```python
from build123d import *

# Parameters (mm, degrees)
F0_W     = 16
F0_H     = 46
F0_R     = 1.65
F0_R_2   = 4
F1_DEPTH = 4
F2_DEPTH = 6.2
F3_DEPTH = 2.2


with BuildPart() as f1:
    # F0 (on Top) → F1 (new body)
    with BuildSketch(Plane.XY):
        Rectangle(F0_W, F0_H)
        with Locations((0, -21)):
            Circle(F0_R, mode=Mode.SUBTRACT)
        with Locations((0, -12)):
            Circle(F0_R_2, mode=Mode.SUBTRACT)
        with Locations((0, 20)):
            Circle(F0_R, mode=Mode.SUBTRACT)
        with Locations((0, 20)):
            Circle(F0_R)
        with Locations((0, -21)):
            Circle(F0_R)
    extrude(amount=F1_DEPTH)

    # F0 (on Top) → F2 (join)
    with BuildSketch(Plane.XY):
        with Locations((0, 20)):
            Circle(F0_R)
        with Locations((0, -21)):
            Circle(F0_R)
    extrude(amount=F2_DEPTH)

    # F0 (on Top) → F3 (cut)
    with BuildSketch(Plane.XY):
        with Locations((0, -21)):
            Circle(F0_R)
        with Locations((0, 20)):
            Circle(F0_R)
    extrude(amount=F3_DEPTH, mode=Mode.SUBTRACT)


solid = f1.part
```
The listing builds one solid part. Answer for the finished solid, in the listing's coordinates (mm). A direction names the side the tool comes from. Round coordinates to 2 decimals unless told otherwise and drop trailing zeros. Loops run counter-clockwise (first coordinate to the right, second up) from the corner with the lowest first, then second, coordinate; pieces in that order, holes last.
Q1. Given pin 1 Ø1 at (x, y) = (-1, 20) entering from -Z; pin 2 Ø1 at (x, y) = (5, -15.5) entering from +Z; pin 3 Ø1.5 at (x, y) = (-1.5, -17.5) entering from -Z, each flat-ended and moving along its own axis, determine where each tip first touches the part or whether it passes through.
Q2. Section C-C, the plane x = 0 is taken. Determine the outline of the cut face in (y, z), then the cut area to 3 significant figures.
Q3. Section A-A, the plane y = -12 is taken. Determine the outline of the cut face in (x, z), then the cut area to 3 significant figures.
Q4. For a pull along Y with two mould halves and no side action, classify faces 4 (the face through (0, 23, 2)), 5 (the face through (0, -23, 2)), 6 (the face through (0, -21, 6.2)), 7 (the face through (-0.215, 21.636, 5.085)) as released by +Y, released by -Y, zero draft, split by the parting line, or undercut.
Q5. Section D-D, the plane z = 3 is taken. Determine the outline of the cut face in (x, y), then the cut area to 3 significant figures.
Q6. Which of the six approach directions +Z, -Z, +X, -X, +Y, -Y give full straight-line access (tool end or side, diameter ignored) to faces 1 (the face through (-0.215, -19.364, 5.085)), 2 (the face through (-0.867, -15.905, 1.972)), 3 (the face through (-0.215, -19.364, 1.085))?
Q7. Section B-B, the plane z = 1 is taken. Determine the outline of the cut face in (x, y).
Q8. Find the intervals of material crossed by line 1 (Y direction, x = 0, z = 0.5); line 2 (Y direction, x = 0, z = 3.15); line 3 (Z direction, x = -5.75, y = 2), in increasing order.
Completed:
1. pin 1: stops at z = 2.2
1. pin 2: stops at z = 4
1. pin 3: stops at z = 0
2. outline: (-23, 0) - (-22.65, 0) - (-22.65, 2.2) - (-19.35, 2.2) - (-19.35, 0) - (-16, 0) - (-16, 4) - (-19.35, 4) - (-19.35, 6.2) - (-22.65, 6.2) - (-22.65, 4) - (-23, 4) - close; (-8, 0) - (18.35, 0) - (18.35, 2.2) - (21.65, 2.2) - (21.65, 0) - (23, 0) - (23, 4) - (21.65, 4) - (21.65, 6.2) - (18.35, 6.2) - (18.35, 4) - (-8, 4) - close
2. area: 152 mm2
3. outline: (-8, 0) - (-4, 0) - (-4, 4) - (-8, 4) - close; (4, 0) - (8, 0) - (8, 4) - (4, 4) - close
3. area: 32.0 mm2
4. face 4: released by +Y
4. face 5: released by -Y
4. face 6: zero draft
4. face 7: undercut
5. outline: (-8, -23) - (8, -23) - (8, 23) - (-8, 23) - close; hole circle Ø8 at (0, -12)
5. area: 686 mm2
6. face 1: +Z
6. face 2: +Z, -Z
6. face 3: -Z
7. outline: (-8, -23) - (8, -23) - (8, 23) - (-8, 23) - close; hole circle Ø8 at (0, -12); hole circle Ø3.3 at (0, -21); hole circle Ø3.3 at (0, 20)
8. line 1: y = -23 to -22.65, -19.35 to -16, -8 to 18.35, 21.65 to 23
8. line 2: y = -23 to -16, -8 to 23
8. line 3: z = 0 to 4
